Check sheet for the modelled part. Datum: model origin and axes. Units: mm. A direction names the side the tool comes from. Give positions to 0.01 mm unless a question says otherwise; leave off trailing zeros. Order: outer loops, then holes, each group sorted by start corner. A loop starts at its lowest first (then second) coordinate and runs counter-clockwise, first axis right, second up. Notation, with made-up numbers: (77.5, 39.25) -> (89.5, 39.25) arc R22 ccw to (89.5, 69.25) -> close; hole circle Ø10 at (49, 53). An arc over 180 degrees is marked (long way). One line per question, with ' | ' between items.
```python
from build123d import *

# Parameters (mm, degrees)
BOX001_W     = 40
BOX001_H     = 40
BOX001_DEPTH = 750
BOX_W        = 50
BOX_H        = 50
BOX_DEPTH    = 750
FILLET_R     = 5
FILLET001_R  = 5


with BuildPart() as box001:
    # Box001 → Box001 (new body)
    with BuildSketch(Plane.XY):
        with Locations((20, 20)):
            Rectangle(BOX001_W, BOX001_H)
    extrude(amount=BOX001_DEPTH)


with BuildPart() as fillet001:
    # Box → Box (new body)
    with BuildSketch(Plane.XY):
        with Locations((25, 25)):
            Rectangle(BOX_W, BOX_H)
    extrude(amount=BOX_DEPTH)

    # Cut: cut Box001
    add(box001.part, mode=Mode.SUBTRACT)

    # Fillet
    fillet_edges = [fillet001.edges().sort_by_distance(p)[0] for p in [
        (40, 0, 375),
    ]]
    fillet(fillet_edges, radius=FILLET_R)

    # Fillet001
    fillet001_edges = [fillet001.edges().sort_by_distance(p)[0] for p in [
        (0, 40, 375),
    ]]
    fillet(fillet001_edges, radius=FILLET001_R)


solid = fillet001.part
```
Q1. Access from +Z, -Z, +X, -X, +Y, -Y to the whole of each face (thin tool, end or side, straight path). Record for faces 1 (the face through (22, 40, 370)), 2 (the face through (25, 50, 370)).
Result sheet:
face 1: +Z, -Z, -X, -Y | face 2: +Z, -Z, +X, -X, +Y
Q2. Thickness scan on line 1 (X direction, y = 19.5, z = 111.5). Record the ranges inside material, lowest first.
Result sheet:
line 1: x = 40 to 50
Q3. Depth check by flat-ended pin: pin 1 Ø5 at (y, z) = (15.5, 442.5) entering from -X; pin 2 Ø10 at (x, z) = (15, 646.5) entering from -Y. Enter the tip coordinate at first touch or a pass-through.
Result sheet:
pin 1: stops at x = 40 | pin 2: stops at y = 40
Q4. Section check B-B (y = 32). Enter the section's corners in (x, z).
Result sheet:
outline: (40, 0) -> (50, 0) -> (50, 750) -> (40, 750) -> close
Q5. Section check A-A (z = 586.5). Enter the section's corners in (x, y).
Result sheet:
outline: (0, 45) arc R5 ccw to (5, 40) -> (40, 40) -> (40, 5) arc R5 ccw to (45, 0) -> (50, 0) -> (50, 50) -> (0, 50) -> close
